Geometry check sheet. Reference: the model listing, model coordinates, mm. Face numbers are marked on the shaded views. A direction names the side the tool comes from. Give positions to 0.01 mm unless a question says otherwise; leave off trailing zeros. Loops run counter-clockwise (first coordinate to the right, second up) from the corner with the lowest first, then second, coordinate; pieces in that order, holes last.
1. Tool access check on the marked faces 1 and 2. Record the directions out of +Z, -Z, +X, -X, +Y, -Y that give a thin tool (end or side, any length) a straight path to the whole face; none if there is none.
2. Material ranges on L1, parallel to X at y = 121, z = 1.75; L2, parallel to Y at x = 145.5, z = -7.75; L3, parallel to Z at x = -22, y = 137.5, recorded low to high.
3. Cross-section at B-B, the plane z = -3.75. Record the cut outline in (x, y), plus the area to 3 significant figures.
4. Cross-section at A-A, the plane y = 127. Record the cut outline in (x, z), plus the area to 3 significant figures.
5. Go/stop test with flat-tipped pins: pin 1 Ø3 at (x, z) = (63, -1) entering from +Y; pin 2 Ø8 at (x, z) = (28.5, -4.5) entering from +Y; pin 3 Ø6 at (x, z) = (101.5, 3) entering from -Y; pin 4 Ø6 at (y, z) = (136, -4.5) entering from -X. Record where each tip stops, or that it passes through.
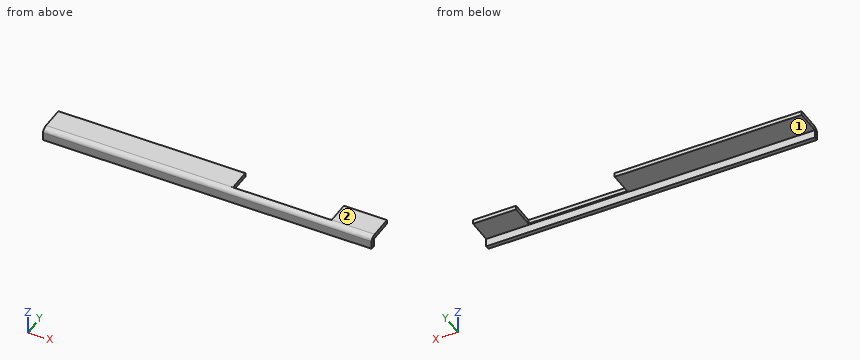
from build123d import *

# Parameters (mm, degrees)
SKETCH_1_W              = 400
SKETCH_1_H              = 35
EXTRUDE_1_DEPTH         = 5
SKETCH_2_W              = 400
SKETCH_2_H              = 5
EXTRUDE_2_DEPTH         = 10
FILLET_1_SIZE           = 7
FILLET_1_SIZE_2         = 5
CUT_EXTRUDE_START       = -5
CUT_EXTRUDE_1_OUTLINE_W = 120
CUT_EXTRUDE_1_OUTLINE_H = 28
CUT_EXTRUDE_1_DEPTH     = 5


# Read off the part's stored shape, not the designer's step: 切除-拉伸1
with BuildPart() as part:
    # 草图1 → 凸台-拉伸1 (new body)
    with BuildSketch(Plane.XY):
        with Locations((32.704402516, 130.419346185)):
            Rectangle(SKETCH_1_W, SKETCH_1_H)
    extrude(amount=EXTRUDE_1_DEPTH)

    # 草图2 → 凸台-拉伸2 (add)
    with BuildSketch(Plane(origin=(0, 0, 0), x_dir=(-1, 0, 0), z_dir=(0, 0, -1))):
        with Locations((-32.704402516, 115.419346185)):
            Rectangle(SKETCH_2_W, SKETCH_2_H)
    extrude(amount=EXTRUDE_2_DEPTH)

    # 圆角1
    # an asymmetric fillet: 7, 5 mm, written as the material it takes off along each edge
    with BuildSketch(Plane(origin=(250.204402516, 112.919346185, 5), x_dir=(0, 1, 0), z_dir=(-1, 0, 0))) as fillet_1_piece_1:
        with BuildLine():
            Bezier((FILLET_1_SIZE, 0), (0, 0), (0, FILLET_1_SIZE_2), weights=[1, 0.707106781, 1])
            Line((0, FILLET_1_SIZE_2), (0, 0))
            Line((0, 0), (FILLET_1_SIZE, 0))
        make_face()
    extrude(amount=435, mode=Mode.SUBTRACT)

    # 切除-拉伸1 outline → 切除-拉伸1 (cut)
    with BuildSketch(Plane.XY.offset(5).offset(CUT_EXTRUDE_START)):
        with Locations((120.204402516, 133.919346185)):
            Rectangle(CUT_EXTRUDE_1_OUTLINE_W, CUT_EXTRUDE_1_OUTLINE_H)
    extrude(amount=CUT_EXTRUDE_1_DEPTH, mode=Mode.SUBTRACT)


solid = part.part
Result:
1. face 1: -Z, +X, -X, +Y
1. face 2: +Z, +X, -X, +Y, -Y
2. L1: x = -167.3 to 60.2, 180.2 to 232.7
2. L2: y = 112.92 to 117.92
2. L3: z = 0 to 5
3. outline: (-167.3, 112.92) - (232.7, 112.92) - (232.7, 117.92) - (-167.3, 117.92) - close
3. area: 2,000 mm2
4. outline: (-167.3, 0) - (60.2, 0) - (60.2, 5) - (-167.3, 5) - close; (180.2, 0) - (232.7, 0) - (232.7, 5) - (180.2, 5) - close
4. area: 1,400 mm2
5. pin 1: stops at y = 119.92
5. pin 2: stops at y = 117.92
5. pin 3: stops at y = 112.92
5. pin 4: passes through
